from build123d import *

# Parameters (mm, degrees)
SKETCH_1_R          = 1.75
EXTRUDE_1_DEPTH     = 3
SKETCH_2_R          = 6
EXTRUDE_2_DEPTH     = 3
SKETCH_3_R          = 1.75
CUT_EXTRUDE_1_DEPTH = 7


with BuildPart() as part:
    # Эскиз1 → Бобышка-Вытянуть1 (new body)
    with BuildSketch(Plane(origin=(0, 0, 0), x_dir=(1, 0, 0), z_dir=(0, 1, 0))):
        with BuildLine():
            Line((-30, 5), (-11.456439237, 5))
            ThreePointArc((-11.456439237, 5), (-10.2750901, 7.118463559), (-8.706840344, 8.968886844))
            ThreePointArc((-8.706840344, 8.968886844), (-8.255178852, 9.942485712), (-8.569645055, 10.968645479))
            Line((-8.569645055, 10.968645479), (-8.619260655, 11.03215055))
            ThreePointArc((-8.619260655, 11.03215055), (8.619260655, 11.03215055), (12.789636407, -5.694313003))
            Line((12.789636407, -5.694313003), (12.716014607, -5.661534466))
            ThreePointArc((12.716014607, -5.661534466), (11.644259912, -5.604659769), (10.808847895, -6.278439868))
            ThreePointArc((10.808847895, -6.278439868), (-0.716551297, -12.47944527), (-11.456439237, -5))
            Line((-11.456439237, -5), (-30, -5))
            ThreePointArc((-30, -5), (-35, 0), (-30, 5))
        make_face()
        with Locations((-30, 0)):
            Circle(SKETCH_1_R, mode=Mode.SUBTRACT)
    extrude(amount=EXTRUDE_1_DEPTH)

    # Эскиз2 → Бобышка-Вытянуть2 (add)
    with BuildSketch(Plane.XZ):
        Circle(SKETCH_2_R)
    extrude(amount=EXTRUDE_2_DEPTH)

    # Эскиз3 → Вырез-Вытянуть1 (cut, through all)
    with BuildSketch(Plane.XZ.offset(3)):
        Circle(SKETCH_3_R)
        with Locations((-7, 0)):
            Circle(SKETCH_3_R)
        with Locations((7, 0)):
            Circle(SKETCH_3_R)
    extrude(amount=-CUT_EXTRUDE_1_DEPTH, mode=Mode.SUBTRACT)


solid = part.part
Design review of the part built by this model. Coordinates are the model's own, in mm. A direction names the side the tool comes from. Round coordinates to 2 decimals unless told otherwise and drop trailing zeros. Write each loop counter-clockwise with the first axis right and the second up, starting at its lowest first coordinate (ties: lowest second). Pieces come first, ordered by that corner, then holes. Notation, with made-up numbers: (72.25, 37.25) - (84.25, 37.25) arc R28 ccw to (84.25, 72.25) - close; hole circle Ø2 at (74.25, 28.5). An arc over 180 degrees is marked (long way). Use a Markdown table: item, result. Add a question column.
1. We need section D-D (z = -4.25). State the section outline as (x, y) points.
2. Mouldability with a two-part tool opening along Z and no side actions: class faces 1 (the face through (0, -1, 6)), 2 (the face through (1.617, -0.042, -0.67)), 3 (the face through (-21, 1, -5)) as +Z half, -Z half, draft (parallel to the pull), parting line (faces both ways), or undercut.
3. For faces 4 (the face through (-10.294, 1.479, -7.09)), 5 (the face through (0, -1, -6)), 6 (the face through (-21, 1, 5)), list the 3-axis set-ups (+Z, -Z, +X, -X, +Y, -Y) from which the entire face can be reached by the end or side of a thin tool; tool diameter is ignored.
4. We need section A-A (z = 0). State the section outline as (x, y) points.
5. We need section B-B (x = 0). State the section outline as (y, z) points.
6. Clearance check with flat-ended pins moving along their axes: pin 1 (1.5 mm diameter, centred on y = -0.5, z = -9.5, fed in from -X); pin 2 (3.5 mm diameter, centred on x = -20, y = 1, fed in from -Z); pin 3 (1.5 mm diameter, centred on y = 0.5, z = 7, fed in from +X). State where each tip first meets the part, or that it passes through.
7. We need section C-C (y = -1.7). State the section outline as (x, z) points, then the cut area to 3 significant figures.
8. Wall thickness on probe 1 along Z at (x, y) = (0, -0.4); probe 2 along Y at (x, z) = (-21, 3); probe 3 along Z at (x, y) = (-31, 1.65): over which ranges is each line inside the solid? List them lowest first.
Output:
| question | item | result |
|---|---|---|
| 1 | outline | (-32.63, 0) - (-4.24, 0) - (-4.24, -3) - (4.24, -3) - (4.24, 0) - (13.34, 0) - (13.34, 3) - (-32.63, 3) - close |
| 2 | face 1 | +Z half |
| 2 | face 2 | undercut |
| 2 | face 3 | -Z half |
| 3 | face 4 | -Z, -X, +Y, -Y |
| 3 | face 5 | -Z, -Y |
| 3 | face 6 | +Z, -X, +Y, -Y |
| 4 | outline | (-35, 0) - (-31.75, 0) - (-31.75, 3) - (-35, 3) - close; (-28.25, 0) - (-8.75, 0) - (-8.75, 3) - (-28.25, 3) - close; (-5.25, -3) - (-1.75, -3) - (-1.75, 3) - (-5.25, 3) - close; (1.75, -3) - (5.25, -3) - (5.25, 3) - (1.75, 3) - close; (8.75, 0) - (14, 0) - (14, 3) - (8.75, 3) - close |
| 5 | outline | (-3, -6) - (0, -6) - (0, -14) - (3, -14) - (3, -1.75) - (-3, -1.75) - close; (-3, 1.75) - (3, 1.75) - (3, 12.5) - (0, 12.5) - (0, 6) - (-3, 6) - close |
| 6 | pin 1 | stops at x = -8.74 |
| 6 | pin 2 | stops at z = -5 |
| 6 | pin 3 | stops at x = 10.83 |
| 7 | outline | (-5.85, -1.32) arc R6 ccw to (5.85, -1.32) arc R1.75 cw to (5.85, 1.32) arc R6 ccw to (-5.85, 1.32) arc R1.75 cw to start; hole circle Ø3.5 at (0, 0) |
| 7 | area | 101 mm2 |
| 8 | probe 1 | z = -6 to -1.75, 1.75 to 6 |
| 8 | probe 2 | y = 0 to 3 |
| 8 | probe 3 | z = -4.9 to -1.44, 1.44 to 4.9 |
